Input: part model. Units: mm. Frame: model coordinates. A direction names the side the tool comes from. Round coordinates to 2 decimals unless told otherwise and drop trailing zeros. Write each loop counter-clockwise with the first axis right and the second up, starting at its lowest first coordinate (ties: lowest second). Pieces come first, ordered by that corner, then holes. Notation, with made-up numbers: (1, 67) - (28, 67) arc R29 cw to (28, 94) - close; hole circle Ø4 at (-15, -16.75). An arc over 180 degrees is marked (long way). Use one line per item in the form item = value.
```python
from build123d import *

# Parameters (mm, degrees)
F0_W     = 19.05
F0_H     = 152.4
F0_W_2   = 152.4
F0_H_2   = 19.05
F1_DEPTH = 19.05


# Not quite as in the source:
# - a feature names something its author has since deleted; it is built from what else it names


with BuildPart() as f1:
    # F0 (on Front) → F1 (new body)
    with BuildSketch(Plane.XZ):
        Polygon((-388.9506477541, -103.6229937509), (-204.8006477541, -103.6229937509), (-204.8006477541, -2.0229937509), (-204.8006477541, 150.3770062491), (-204.8006477541, 201.1770062491), (-725.5006477541, 201.1770062491), (-725.5006477541, 150.3770062491), (-725.5006477541, -2.0229937509), (-725.5006477541, -103.6229937509), (-541.3506477541, -103.6229937509), align=None)
        with Locations((-735.0256477541, 74.1770062491)):
            Rectangle(F0_W, F0_H)
        with Locations((-195.2756477541, 74.1770062491)):
            Rectangle(F0_W, F0_H)
        with Locations((-465.1506477541, -113.1479937509)):
            Rectangle(F0_W_2, F0_H_2)
    extrude(amount=F1_DEPTH)


solid = f1.part
```
(1) Cut plane B-B on x = -626. Output: boundary loops of the cut face in (y, z), then the cut area to 3 significant figures.
Derived:
outline = (-19.05, -103.62) - (0, -103.62) - (0, 201.18) - (-19.05, 201.18) - close
area = 5,810 mm^2
(2) Material intervals for L1, parallel to Z at x = -710.5, y = -2.25; L2, parallel to X at y = -4.75, z = 152, sorted ascending.
Derived:
L1 = -103.62 to 201.18
L2 = -725.5 to -204.8
(3) Cut plane C-C on z = -98. Output: boundary loops of the cut face in (x, y).
Derived:
outline = (-725.5, -19.05) - (-204.8, -19.05) - (-204.8, 0) - (-725.5, 0) - close
(4) Cut plane A-A on y = -5.5. Output: boundary loops of the cut face in (x, z), then the cut area to 3 significant figures.
Derived:
outline = (-744.55, -2.02) - (-725.5, -2.02) - (-725.5, -103.62) - (-541.35, -103.62) - (-541.35, -122.67) - (-388.95, -122.67) - (-388.95, -103.62) - (-204.8, -103.62) - (-204.8, -2.02) - (-185.75, -2.02) - (-185.75, 150.38) - (-204.8, 150.38) - (-204.8, 201.18) - (-725.5, 201.18) - (-725.5, 150.38) - (-744.55, 150.38) - close
area = 167,000 mm^2
(5) Draft query along X for faces 1 (the face through (-204.801, -9, 175)), 2 (the face through (-195, -9, -2.023)), 3 (the face through (-725.501, -9, -52)). Return one class per face: released by +X, released by -X, zero draft, split by the parting line, or undercut.
Derived:
face_1 = released by +X
face_2 = zero draft
face_3 = released by -X
(6) First-contact query: pin 1 Ø5.5 at (x, y) = (-255.5, -6.5) entering from -Z; pin 2 Ø9.5 at (x, y) = (-732, -12) entering from +Z; pin 3 Ø3 at (y, z) = (-5, -89) entering from +X. Flat tips, straight axial feed; report the tip coordinate or a pass-through.
Derived:
pin_1 = -103.62
pin_2 = 150.38
pin_3 = -204.8
(7) Access query for faces 4 (the face through (-735, -9, 150.377)), 5 (the face through (-195, -9, 150.377)), 6 (the face through (-185.751, -9, 73)), 7 (the face through (-204.801, -9, -54)), 8 (the face through (-635, -9, -103.623)). Directions: +Z, -Z, +X, -X, +Y, -Y. A direction counts if a zero-diameter tool reaches every point of the face in a straight line with its end or side. Return the directions, or none.
Derived:
face_4 = +Z, -X, +Y, -Y
face_5 = +Z, +X, +Y, -Y
face_6 = +Z, -Z, +X, +Y, -Y
face_7 = -Z, +X, +Y, -Y
face_8 = -Z, -X, +Y, -Y
